Source: CAD feature listing. Evaluate the final solid. Frame: model axes, mm. A direction names the side the tool comes from. Round coordinates to 2 decimals unless told otherwise and drop trailing zeros. Loops run counter-clockwise (first coordinate to the right, second up) from the corner with the lowest first, then second, coordinate; pieces in that order, holes last. Notation, with made-up numbers: (12.5, 13.5) - (48.5, 13.5) arc R19 ccw to (48.5, 17.5) - close; hole circle Ø7 at (43, -11). An arc over 180 degrees is marked (long way). Use CSV: the item, a comma, the result in double quotes. Start each with the question number.
from build123d import *

# Parameters (mm, degrees)
F1_DEPTH = 927.1
F3_DEPTH = 850.9
F4_W     = 139.7
F4_H     = 254
F5_DEPTH = 850.9


with BuildPart() as f1:
    # F0 (on Right) → F1 (new body, symmetric)
    with BuildSketch(Plane.YZ):
        Polygon((-658.550496, 596.9), (-658.550496, 0), (319.349504, 0), (357.449504, 596.9), align=None)
    extrude(amount=F1_DEPTH, both=True)

    # F2 (on Right) → F3 (cut, symmetric)
    with BuildSketch(Plane.YZ):
        Polygon((-658.550496, 596.9), (-658.550496, 254), (217.749504, 254), (255.849504, 596.9), align=None)
    extrude(amount=F3_DEPTH, both=True, mode=Mode.SUBTRACT)

    # F4 (on Right) → F5 (join, symmetric)
    with BuildSketch(Plane.YZ):
        with Locations((-728.400496, 127)):
            Rectangle(F4_W, F4_H)
    extrude(amount=F5_DEPTH, both=True)


solid = f1.part
1. Section query C-C on z = 359. Return the cut outline in (x, y), and give its area (3 significant figures).
2. Contact query for flat-ended pins moving along their axis: P1, Ø12, axis at x = -398, y = -283.5, coming from the +Z side; P2, Ø12, axis at x = 399.5, z = 178.5, coming from the +Y side; P3, Ø1.5, axis at x = 353, z = 439.5, coming from the -Y side. Output: stop coordinate, or through.
3. Line query: line 1 along X through (y, z) = (-458, 520.5); line 2 along Z through (x, y) = (428, -66); line 3 along Y through (x, z) = (215.5, 427). Output: solid intervals per line, ascending.
4. Reachability of faces 5 (the flat face through (-888, -658.55, 303)), 6 (the flat face through (850.9, -208, 428)), 7 (the flat face through (850.9, -729, 129)) from +Z, -Z, +X, -X, +Y, -Y: full face, straight path, thin tool, end or side. Return the list, or none.
5. Mould query, pull axis X, two halves, no side actions, for faces 1 (the flat face through (12.979, 338.133, 294.272)), 2 (the flat face through (927.1, -158, 303)), 3 (the flat face through (12, -297, 254)), 4 (the flat face through (11.913, 236.533, 423.05)). Classes: +X half, -X half, draft (parallel to the pull), parting line (faces both ways), or undercut.
6. Section query A-A on x = -302.5. Return the cut outline in (y, z).
7. Section query D-D on y = -686.5. Return the cut outline in (x, z).
8. Section query B-B on y = -30.5. Return the cut outline in (x, z), and give its area (3 significant figures).
Values:
1,outline,"(-927.1, -658.55) - (-850.9, -658.55) - (-850.9, 229.42) - (850.9, 229.42) - (850.9, -658.55) - (927.1, -658.55) - (927.1, 342.26) - (-927.1, 342.26) - close"
1,area,"345,000 mm^2"
2,P1,"stops at z = 254"
2,P2,"stops at y = 331.13"
2,P3,"stops at y = 238.28"
3,line 1,"x = -927.1 to -850.9, 850.9 to 927.1"
3,line 2,"z = 0 to 254"
3,line 3,"y = 236.97 to 346.6"
4,face 5,"+Z, -Z, -X, -Y"
4,face 6,"+Z, -Y"
4,face 7,"+Z, -Z, +X, -Y"
5,face 1,"draft"
5,face 2,"+X half"
5,face 3,"undercut"
5,face 4,"undercut"
6,outline,"(-798.25, 0) - (319.35, 0) - (357.45, 596.9) - (255.85, 596.9) - (217.75, 254) - (-798.25, 254) - close"
7,outline,"(-850.9, 0) - (850.9, 0) - (850.9, 254) - (-850.9, 254) - close"
8,outline,"(-927.1, 0) - (927.1, 0) - (927.1, 596.9) - (850.9, 596.9) - (850.9, 254) - (-850.9, 254) - (-850.9, 596.9) - (-927.1, 596.9) - close"
8,area,"523,000 mm^2"
